```python
from build123d import *

# Parameters (mm, degrees)
SKETCH_1_R      = 18.68
SKETCH_1_R_2    = 15.652173913
EXTRUDE_2_DEPTH = 2
SKETCH_1_4_R    = 23
SKETCH_1_4_R_2  = 1.25
SKETCH_1_4_R_3  = 18.68
EXTRUDE_3_DEPTH = 8


with BuildPart() as part:
    # 草图1 → 凸台-拉伸2 (new body)
    with BuildSketch(Plane(origin=(0, 0, 0), x_dir=(0, 0, -1), z_dir=(1, 0, 0))):
        Circle(SKETCH_1_R)
        Circle(SKETCH_1_R_2, mode=Mode.SUBTRACT)
    extrude(amount=EXTRUDE_2_DEPTH)

    # 草图1<4> → 凸台-拉伸3 (add)
    with BuildSketch(Plane(origin=(0, 0, 0), x_dir=(0, 0, -1), z_dir=(1, 0, 0))):
        Circle(SKETCH_1_4_R)
        with Locations((-7.940681222, 19.1705003)):
            Circle(SKETCH_1_4_R_2, mode=Mode.SUBTRACT)
        with Locations((-19.1705003, 7.940681222)):
            Circle(SKETCH_1_4_R_2, mode=Mode.SUBTRACT)
        with Locations((-19.1705003, -7.940681222)):
            Circle(SKETCH_1_4_R_2, mode=Mode.SUBTRACT)
        with Locations((-7.940681222, -19.1705003)):
            Circle(SKETCH_1_4_R_2, mode=Mode.SUBTRACT)
        with Locations((7.940681222, -19.1705003)):
            Circle(SKETCH_1_4_R_2, mode=Mode.SUBTRACT)
        with Locations((19.1705003, -7.940681222)):
            Circle(SKETCH_1_4_R_2, mode=Mode.SUBTRACT)
        with Locations((19.1705003, 7.940681222)):
            Circle(SKETCH_1_4_R_2, mode=Mode.SUBTRACT)
        with Locations((7.940681222, 19.1705003)):
            Circle(SKETCH_1_4_R_2, mode=Mode.SUBTRACT)
        Circle(SKETCH_1_4_R_3, mode=Mode.SUBTRACT)
    extrude(amount=EXTRUDE_3_DEPTH)


solid = part.part
```
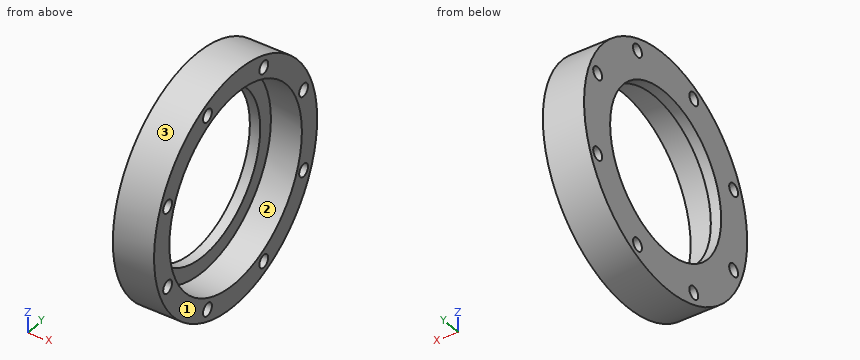
Could you check a few things on this model? Use its own coordinates, in mm. Face numbers are marked on the shaded views. Give positions to 0.01 mm unless a question says otherwise; leave off trailing zeros. Loops run counter-clockwise (first coordinate to the right, second up) from the corner with the lowest first, then second, coordinate; pieces in that order, holes last. Notation, with made-up numbers: (61.5, 17.25) - (86.5, 17.25) arc R18 ccw to (86.5, 23.25) - close; hole circle Ø9 at (37, -2). An arc over 180 degrees is marked (long way). Answer in a Markdown table with one row per item. Add a question column.
Q1. If we section it at A-A (y = 0): List the corners of the cut face in (x, z) for me.
Q2. If we section it at C-C (x = 0.75): State how many separate pieces and enclosed holes the cut face has, plus the area to 3 significant figures.
Q3. Please list where these lines run through material, in increasing order: L1, parallel to Z at x = 0.75, y = -7.5; L2, parallel to Z at x = 2.25, y = 19.5; L3, parallel to Z at x = 4, y = -7. Write a range as from..to.
Q4. For pin 1 (1.5 mm diameter, centred on y = -19.17, z = 7.94, fed in from -X); pin 2 (1.5 mm diameter, centred on x = 7, y = -9.5, fed in from -Z); pin 3 (1 mm diameter, centred on x = 5.5, y = 12, fed in from +Z), each with a flat end and sliding along its axis, tell me the tip position at first contact or that it passes through.
Q5. We'd pull the mould along Z, two halves only. Please class the marked faces 1, 2 and 3: +Z half, -Z half, draft (parallel to the pull), parting line (faces both ways), or undercut.
The answers:
| question | item | result |
|---|---|---|
| 1 | outline | (0, -23) - (8, -23) - (8, -18.68) - (2, -18.68) - (2, -15.65) - (0, -15.65) - close; (0, 15.65) - (2, 15.65) - (2, 18.68) - (8, 18.68) - (8, 23) - (0, 23) - close |
| 2 | separate pieces | 1 |
| 2 | enclosed holes | 9 |
| 2 | area | 853 mm^2 |
| 3 | L1 | z = -21.74..-20.34, -18..-13.74, 13.74..18, 20.34..21.74 |
| 3 | L2 | z = -12.2..-9.15, -6.73..6.73, 9.15..12.2 |
| 3 | L3 | z = -21.91..-19.99, -18.35..-17.32, 17.32..18.35, 19.99..21.91 |
| 4 | pin 1 | passes through |
| 4 | pin 2 | stops at z = -21.27 |
| 4 | pin 3 | stops at z = 19.92 |
| 5 | face 1 | draft |
| 5 | face 2 | undercut |
| 5 | face 3 | parting line |
